Could you check a few things on this drawing? It's one solid part, dimensions in mm from its lowest x, y, z. A direction names the side the tool comes from. Round coordinates to 2 decimals unless told otherwise and drop trailing zeros. Order: outer loops, then holes, each group sorted by start corner. A loop starts at its lowest first (then second) coordinate and runs counter-clockwise, first axis right, second up.
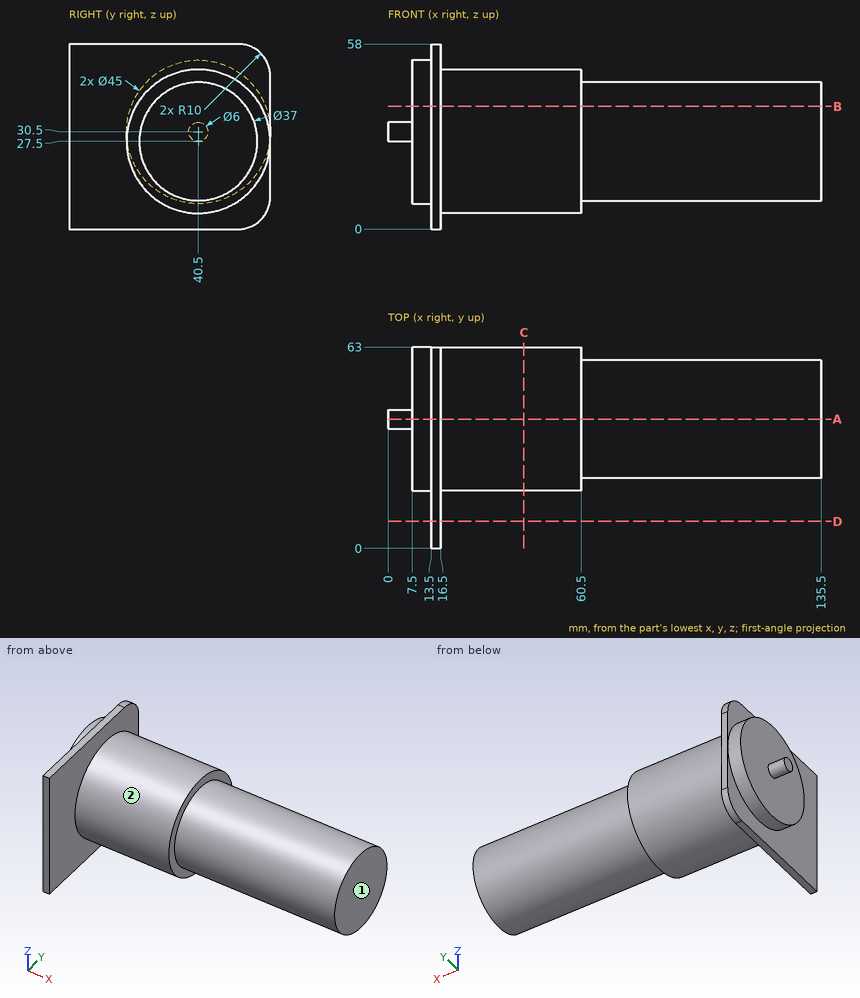
1) I need wall thicknesses on line 1 (X direction, y = 25, z = 32); line 2 (Y direction, x = 74, z = 28); line 3 (X direction, y = 7, z = 26). Which ranges of each line are inside material? Lowest first, please.
2) If we section it at A-A (y = 40.5): Write out the boundary of the cut face in (x, z), plus the area to 3 significant figures.
3) I'm going to push flat-ended pins straight in: pin 1 (10 mm diameter, centred on x = 19.5, y = 30, fed in from +Z); pin 2 (1.5 mm diameter, centred on x = 88.5, z = 21, fed in from -Y); pin 3 (2 mm diameter, centred on x = 55.5, y = 38.5, fed in from -Z); pin 4 (1 mm diameter, centred on x = 59, z = 38, fed in from +Y). Where does each tip first touch, or does it pass through?
4) If we section it at B-B (z = 38.5): Write out the boundary of the cut face in (x, y).
5) If we section it at D-D (y = 8.5): Write out the boundary of the cut face in (x, z), plus the area to 3 significant figures.
6) If we section it at C-C (x = 42.5): Write out the boundary of the cut face in (y, z), plus the area to 3 significant figures.
7) For the marked faces 1 and 2, which set-ups out of +Z, -Z, +X, -X, +Y, -Y let a thin tool reach every point of the face, with its end or its side?
Solutions:
1. line 1: x = 7.5 to 135.5
1. line 2: y = 22.01 to 58.99
1. line 3: x = 13.5 to 16.5
2. outline: (0, 27.5) - (7.5, 27.5) - (7.5, 8) - (13.5, 8) - (13.5, 0) - (16.5, 0) - (16.5, 5) - (60.5, 5) - (60.5, 9) - (135.5, 9) - (135.5, 46) - (60.5, 46) - (60.5, 50) - (16.5, 50) - (16.5, 58) - (13.5, 58) - (13.5, 53) - (7.5, 53) - (7.5, 33.5) - (0, 33.5) - close
2. area: 5,240 mm2
3. pin 1: stops at z = 58
3. pin 2: stops at y = 22.92
3. pin 3: stops at z = 5.02
3. pin 4: stops at y = 60.66
4. outline: (7.5, 19.47) - (13.5, 19.47) - (13.5, 0) - (16.5, 0) - (16.5, 20.87) - (60.5, 20.87) - (60.5, 25.63) - (135.5, 25.63) - (135.5, 55.37) - (60.5, 55.37) - (60.5, 60.13) - (16.5, 60.13) - (16.5, 63) - (13.5, 63) - (13.5, 61.53) - (7.5, 61.53) - close
5. outline: (13.5, 0) - (16.5, 0) - (16.5, 58) - (13.5, 58) - close
5. area: 174 mm2
6. outline: circle Ø45 at (40.5, 27.5)
6. area: 1,590 mm2
7. face 1: +Z, -Z, +X, +Y, -Y
7. face 2: +X
